Part model, mm, in its own coordinate system. Give positions to 0.01 mm unless a question says otherwise; leave off trailing zeros. Loops run counter-clockwise (first coordinate to the right, second up) from the corner with the lowest first, then second, coordinate; pieces in that order, holes last. Notation, with made-up numbers: M 63,61.5 L 71,61.5 A21 ccw 71,66.5 Z; hole C 88,-7 d10. An arc over 180 degrees is marked long. Answer in a Markdown table with one row per item.
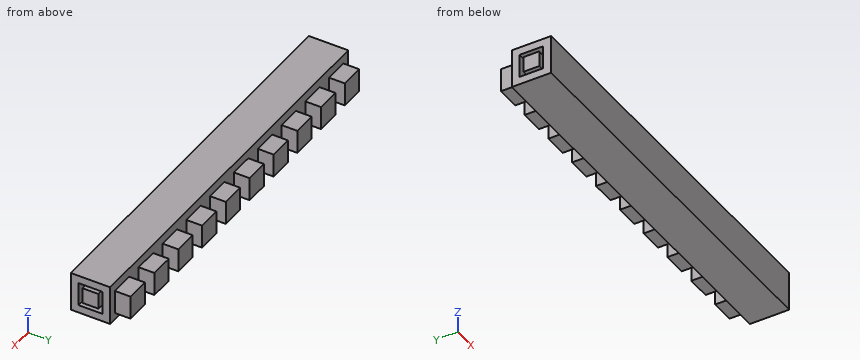
from build123d import *

# Parameters (mm, degrees)
F0_W     = 50
F0_H     = 5
F1_DEPTH = 5
F2_W     = 3
F2_H     = 3
F3_DEPTH = 2
F4_W     = 3
F4_H     = 3
F4_W_2   = 2
F4_H_2   = 2
F5_DEPTH = 3
F6_W     = 3
F6_H     = 3
F6_W_2   = 2
F6_H_2   = 2
F7_DEPTH = 3


with BuildPart() as f1:
    # F0 (on Front) → F1 (new body)
    with BuildSketch(Plane.XZ):
        with Locations((-10.476069, 8.731769)):
            Rectangle(F0_W, F0_H)
    extrude(amount=F1_DEPTH)

    # F2 (on Front) → F3 (join)
    with BuildSketch(Plane.XZ):
        with Locations((-32.976069, 8.585279)):
            Rectangle(F2_W, F2_H)
        with Locations((-27.976069, 8.585279)):
            Rectangle(F2_W, F2_H)
        with Locations((-22.976069, 8.585279)):
            Rectangle(F2_W, F2_H)
        with Locations((-17.976069, 8.585279)):
            Rectangle(F2_W, F2_H)
        with Locations((-12.976069, 8.585279)):
            Rectangle(F2_W, F2_H)
        with Locations((-7.976069, 8.585279)):
            Rectangle(F2_W, F2_H)
        with Locations((-2.976069, 8.585279)):
            Rectangle(F2_W, F2_H)
        with Locations((2.023931, 8.585279)):
            Rectangle(F2_W, F2_H)
        with Locations((7.023931, 8.585279)):
            Rectangle(F2_W, F2_H)
        with Locations((12.023931, 8.585279)):
            Rectangle(F2_W, F2_H)
    extrude(amount=-F3_DEPTH)

    # F4 (on face) → F5 (cut)
    with BuildSketch(Plane(origin=(-35.476069, 0, 0), x_dir=(0, -1, 0), z_dir=(-1, 0, 0))):
        with Locations((2.5, 8.731769)):
            Rectangle(F4_W, F4_H)
        with Locations((2.5, 8.731769)):
            Rectangle(F4_W_2, F4_H_2, mode=Mode.SUBTRACT)
    extrude(amount=-F5_DEPTH, mode=Mode.SUBTRACT)

    # F6 (on face) → F7 (cut)
    with BuildSketch(Plane.YZ.offset(14.523931)):
        with Locations((-2.5, 8.731769)):
            Rectangle(F6_W, F6_H)
        with Locations((-2.5, 8.731769)):
            Rectangle(F6_W_2, F6_H_2, mode=Mode.SUBTRACT)
    extrude(amount=-F7_DEPTH, mode=Mode.SUBTRACT)


solid = f1.part
(1) Drill centre lines: line 1 along Y through (x, z) = (-27, 7.05); line 2 along X through (y, z) = (-3.75, 7.5). Where is each one in solid material? Low to high.
Recorded:
| item | result |
|---|---|
| line 1 | y = -5 to 0 |
| line 2 | x = -32.48 to 11.52 |
(2) Saw through at A-A (y = 1). Give the number of separate pieces and of enclosed holes in the cut face, plus the area to 3 significant figures.
Recorded:
| item | result |
|---|---|
| separate pieces | 10 |
| enclosed holes | 0 |
| area | 90.0 mm^2 |
(3) Saw through at B-B (x = -8). Write the cut outline in (y, z), plus the area to 3 significant figures.
Recorded:
| item | result |
|---|---|
| outline | M -5,6.23 L 0,6.23 L 0,7.09 L 2,7.09 L 2,10.09 L 0,10.09 L 0,11.23 L -5,11.23 Z |
| area | 31.0 mm^2 |
(4) Saw through at D-D (z = 6.65). Write the cut outline in (x, y), plus the area to 3 significant figures.
Recorded:
| item | result |
|---|---|
| outline | M -35.48,-5 L 14.52,-5 L 14.52,0 L -35.48,0 Z |
| area | 250 mm^2 |
(5) Pin check, flat tips, straight feed: pin 1 Ø1 at (x, y) = (7, 1) entering from +Z; pin 2 Ø1.6 at (y, z) = (0.5, 8.5) entering from +X; pin 3 Ø0.6 at (x, y) = (-23, 1) entering from -Z; pin 4 Ø0.6 at (y, z) = (0.5, 8) entering from +X. Stop position of each tip, or through.
Recorded:
| item | result |
|---|---|
| pin 1 | stops at z = 10.09 |
| pin 2 | stops at x = 14.52 |
| pin 3 | stops at z = 7.09 |
| pin 4 | stops at x = 13.52 |
(6) Saw through at C-C (y = -2.5). Write the cut outline in (x, z), plus the area to 3 significant figures.
Recorded:
| item | result |
|---|---|
| outline | M -35.48,6.23 L 14.52,6.23 L 14.52,7.23 L 11.52,7.23 L 11.52,7.73 L 14.52,7.73 L 14.52,9.73 L 11.52,9.73 L 11.52,10.23 L 14.52,10.23 L 14.52,11.23 L -35.48,11.23 L -35.48,10.23 L -32.48,10.23 L -32.48,9.73 L -35.48,9.73 L -35.48,7.73 L -32.48,7.73 L -32.48,7.23 L -35.48,7.23 Z |
| area | 244 mm^2 |
